CAD build for the part. Positions are in the model's coordinates, mm. A direction names the side the tool comes from. Round coordinates to 2 decimals unless told otherwise and drop trailing zeros. Loops run counter-clockwise (first coordinate to the right, second up) from the corner with the lowest first, then second, coordinate; pieces in that order, holes last.
from build123d import *

# Parameters (mm, degrees)
SKETCH1_R               = 125
BOSS_EXTRUDE1_DEPTH     = 100
FILLET1_R               = 20
SKETCH2_R               = 11.805832703
CUT_EXTRUDE1_DEPTH      = 126
CUT_EXTRUDE1_DEPTH_BACK = 126
SKETCH3_R               = 75
BOSS_EXTRUDE2_DEPTH     = 100
CHAMFER1_SIZE           = 28.26
CHAMFER1_SIZE2          = 16.980321094


with BuildPart() as part:
    # Sketch1 → Boss-Extrude1 (new body)
    with BuildSketch(Plane.XY):
        Circle(SKETCH1_R)
    extrude(amount=BOSS_EXTRUDE1_DEPTH)

    # Fillet1
    fillet1_edges = [part.edges().sort_by_distance(p)[0] for p in [
        (-125, 0, 100),
    ]]
    fillet(fillet1_edges, radius=FILLET1_R)

    # Sketch2 → Cut-Extrude1 (cut, two sides)
    with BuildSketch(Plane(origin=(0, 0, 0), x_dir=(1, 0, 0), z_dir=(0, 1, 0))) as cut_extrude1_sk:
        with Locations((-46.950776643, -80)):
            Circle(SKETCH2_R)
        with BuildLine():
            Line((16.547286213, -71.022688997), (45.520734854, -71.022688997))
            ThreePointArc((45.520734854, -71.022688997), (54.498045857, -80), (45.520734854, -88.977311003))
            Line((45.520734854, -88.977311003), (16.547286213, -88.977311003))
            ThreePointArc((16.547286213, -88.977311003), (7.56997521, -80), (16.547286213, -71.022688997))
        make_face()
    extrude(amount=CUT_EXTRUDE1_DEPTH, mode=Mode.SUBTRACT)
    extrude(cut_extrude1_sk.sketch, amount=-CUT_EXTRUDE1_DEPTH_BACK, mode=Mode.SUBTRACT)

    # Sketch3 → Boss-Extrude2 (add)
    with BuildSketch(Plane(origin=(0, 0, 0), x_dir=(-1, 0, 0), z_dir=(0, 0, -1))):
        Circle(SKETCH3_R)
    extrude(amount=BOSS_EXTRUDE2_DEPTH)

    # Chamfer1
    chamfer1_edges = [part.edges().sort_by_distance(p)[0] for p in [
        (75, 0, 0),
    ]]
    chamfer1_side = [part.faces().sort_by_distance(p)[0] for p in [
        (-121.464466094, 0, 0),
    ]]
    chamfer(chamfer1_edges, length=CHAMFER1_SIZE, length2=CHAMFER1_SIZE2, reference=chamfer1_side[0])


solid = part.part
Item 1: Cut at B-B (z = 29.5). List the corners of the cut face in (x, y).
Verdict:
outline: circle Ø250 at (0, 0)
Item 2: Flat gauge pins, fed straight in: P1, Ø1.5, axis at x = 59, z = 36, coming from the -Y side; P2, Ø6, axis at x = 56, z = 77, coming from the -Y side (3 decimals); P3, Ø5, axis at x = -54.5, z = -55, coming from the +Y side. Where does each tip first touch, or does it go through?
Verdict:
P1: stops at y = -110.6
P2: stops at y = -113.045
P3: stops at y = 54.05
Item 3: Wall check: L1, parallel to X at y = 29, z = 80; L2, parallel to X at y = 58, z = 80; L3, parallel to Z at x = 43, y = 94.5. Give the ranges that are in metal, low to high.
Verdict:
L1: x = -121.59 to -58.76, -35.14 to 7.57, 54.5 to 121.59
L2: x = -110.73 to -58.76, -35.14 to 7.57, 54.5 to 110.73
L3: z = 0 to 71.02, 88.98 to 100
Item 4: Cut at A-A (x = 0). List the corners of the cut face in (y, z).
Verdict:
outline: (-125, 0) - (-103.26, 0) - (-75, -16.98) - (-75, -100) - (75, -100) - (75, -16.98) - (103.26, 0) - (125, 0) - (125, 80) arc R20 ccw to (105, 100) - (-105, 100) arc R20 ccw to (-125, 80) - close
Item 5: Cut at C-C (y = 39.5). State how many separate pieces and enclosed holes the cut face has, plus the area to 3 significant figures.
Verdict:
separate pieces: 1
enclosed holes: 2
area: 35,600 mm2
Item 6: 3-axis set-ups, long thin cutter, end or side, ignore diameter. For faces 1 (the cylindrical face through (-124.88, 5.5, 39.44)), 2 (the cylindrical face through (9.764, 74.362, -57.909)): which of +Z, -Z, +X, -X, +Y, -Y reach the whole face in a straight line?
Verdict:
face 1: +Z, -Z
face 2: -Z
